Build history of the part. All positions in model axes, mm. A direction names the side the tool comes from. Round coordinates to 2 decimals unless told otherwise and drop trailing zeros. Loops run counter-clockwise (first coordinate to the right, second up) from the corner with the lowest first, then second, coordinate; pieces in that order, holes last. Notation, with made-up numbers: M 24.25,83.25 L 43.25,83.25 A29 ccw 43.25,116.25 Z; hole C -0.75,13 d4. An arc over 180 degrees is marked long. Use one line per item in the form item = value. Start each with the question number.
```python
from build123d import *

# Parameters (mm, degrees)
F0_R      = 12.5
F0_R_2    = 11.5
F1_DEPTH  = 8
F3_R      = 4
F4_DEPTH  = 8.001
F2_R      = 11.0174189911
F5_DEPTH  = 1
F6_R      = 5
F6_R_2    = 4
F7_DEPTH  = 1
F9_R      = 270.8400585349
F9_R_2    = 127
F10_DEPTH = 1
F11_R     = 11.5
F11_R_2   = 5
F12_DEPTH = 1


with BuildPart() as f1:
    # F0 (on Top) → F1 (new body)
    with BuildSketch(Plane.XY):
        Circle(F0_R)
        Circle(F0_R_2, mode=Mode.SUBTRACT)
        Circle(F0_R_2)
    extrude(amount=F1_DEPTH)

    # F3 (on face) → F4 (cut, through all)
    with BuildSketch(Plane.XY.offset(8)):
        Circle(F3_R)
    extrude(amount=-F4_DEPTH, mode=Mode.SUBTRACT)

    # F2 (on face) → F5 (cut)
    with BuildSketch(Plane.XY.offset(8)):
        Circle(F2_R)
    extrude(amount=-F5_DEPTH, mode=Mode.SUBTRACT)

    # F6 (on face) → F7 (join)
    with BuildSketch(Plane.XY.offset(7)):
        Circle(F6_R)
        Circle(F6_R_2, mode=Mode.SUBTRACT)
    extrude(amount=F7_DEPTH)

    # F9 (on face) → F10 (cut)
    with BuildSketch(Plane(origin=(0, 0, 0), x_dir=(1, 0, 0), z_dir=(0, 0, -1))):
        Circle(F9_R)
        Circle(F9_R_2, mode=Mode.SUBTRACT)
    extrude(amount=-F10_DEPTH, mode=Mode.SUBTRACT)

    # F11 (on face) → F12 (cut)
    with BuildSketch(Plane(origin=(0, 0, 0), x_dir=(1, 0, 0), z_dir=(0, 0, -1))):
        Circle(F11_R)
        Circle(F11_R_2, mode=Mode.SUBTRACT)
    extrude(amount=-F12_DEPTH, mode=Mode.SUBTRACT)


solid = f1.part
```
Q1. Drop flat-ended pins along their axis: P1, Ø1, axis at y = -6, z = 3, coming from the +X side (3 decimals); P2, Ø1, axis at x = -4, z = 2, coming from the +Y side; P3, Ø2, axis at y = 3.5, z = 6.5, coming from the +X side. Give the stop position or say it passes through.
Q2. Saw through at D-D (x = 6.25). Give the cut face in (y, z), and give its area (3 significant figures).
Q3. Saw through at C-C (y = -9.75). Give the cut face in (x, z), and give its area (3 significant figures).
Q4. Saw through at B-B (x = -2.25). Give the cut face in (y, z), and give its area (3 significant figures).
Q5. Wall check: probe 1 along Y at (x, z) = (0, 7.4); probe 2 along Y at (x, z) = (0, 0.65); probe 3 along Y at (x, z) = (0, 3). Give the ranges that are in metal, low to high.
Q6. Tool access for faces 1 (the face through (11, -4, 0)), 2 (the face through (-1.08, -4.88, 7.49)), 3 (the face through (-1.08, 4.88, 0.49)): list every direction of +Z, -Z, +X, -X, +Y, -Y with a clear straight run to the whole face (end or side of a thin tool).
Q7. Saw through at A-A (y = 0). Give the cut face in (x, z).
Q8. Pull direction Y, two halves, no side cores. Call faces 4 (the face through (-8.12, 7.446, 7.507)), 5 (the face through (5, -10, 8)), 6 (the face through (11.923, 3.755, 3.944)): pulls with the +Y half, pulls with the -Y half, needs draft (parallel to the pull), parting line crosses it, or undercut.
Filled in:
q1.P1 = 11.225
q1.P2 = 12
q1.P3 = 12.25
q2.outline = M -10.83,0 L -9.65,0 L -9.65,1 L 9.65,1 L 9.65,0 L 10.83,0 L 10.83,8 L 9.07,8 L 9.07,7 L -9.07,7 L -9.07,8 L -10.83,8 Z
q2.area = 136 mm²
q3.outline = M -7.82,0 L -6.1,0 L -6.1,1 L 6.1,1 L 6.1,0 L 7.82,0 L 7.82,8 L 5.13,8 L 5.13,7 L -5.13,7 L -5.13,8 L -7.82,8 Z
q3.area = 103 mm²
q4.outline = M -12.3,0 L -11.28,0 L -11.28,1 L -4.47,1 L -4.47,0 L -3.31,0 L -3.31,8 L -4.47,8 L -4.47,7 L -10.79,7 L -10.79,8 L -12.3,8 Z; M 3.31,0 L 4.47,0 L 4.47,1 L 11.28,1 L 11.28,0 L 12.3,0 L 12.3,8 L 10.79,8 L 10.79,7 L 4.47,7 L 4.47,8 L 3.31,8 Z
q4.area = 118 mm²
q5.probe_1 = -12.5 to -11.02, -5 to -4, 4 to 5, 11.02 to 12.5
q5.probe_2 = -12.5 to -11.5, -5 to -4, 4 to 5, 11.5 to 12.5
q5.probe_3 = -12.5 to -4, 4 to 12.5
q6.face_1 = -Z, +X, -X, +Y, -Y
q6.face_2 = +Z
q6.face_3 = -Z
q7.outline = M -12.5,0 L -11.5,0 L -11.5,1 L -5,1 L -5,0 L -4,0 L -4,8 L -5,8 L -5,7 L -11.02,7 L -11.02,8 L -12.5,8 Z; M 4,0 L 5,0 L 5,1 L 11.5,1 L 11.5,0 L 12.5,0 L 12.5,8 L 11.02,8 L 11.02,7 L 5,7 L 5,8 L 4,8 Z
q8.face_4 = undercut
q8.face_5 = needs draft
q8.face_6 = parting line crosses it
